Here's how the part is built. I have some questions about the finished solid (model axes, mm). Give positions to 0.01 mm unless a question says otherwise; leave off trailing zeros. Order: outer loops, then holes, each group sorted by start corner. A loop starts at its lowest first (then second) coordinate and runs counter-clockwise, first axis right, second up. Notation, with made-up numbers: M -36.5,44.25 L -17.5,44.25 A27 cw -17.5,77.25 Z; hole C 34,1 d1. An arc over 180 degrees is marked long. Use one line per item in the form item = value.
from build123d import *

# Parameters (mm, degrees)
SKETCH1_R           = 2
BOSS_EXTRUDE1_DEPTH = 50


with BuildPart() as part:
    # Sketch1 → Boss-Extrude1 (new body)
    with BuildSketch(Plane.XY):
        with BuildLine():
            Line((3.9, 2.839339828), (5.451585007, 4.390924835))
            ThreePointArc((5.451585007, 4.390924835), (4.949747468, 4.949747468), (4.390924835, 5.451585007))
            Line((4.390924835, 5.451585007), (2.839339828, 3.9))
            Line((2.839339828, 3.9), (0.519615242, 3.9))
            Line((0.519615242, 3.9), (0, 3.6))
            Line((0, 3.6), (-0.519615242, 3.9))
            Line((-0.519615242, 3.9), (-2.839339828, 3.9))
            Line((-2.839339828, 3.9), (-4.390924835, 5.451585007))
            ThreePointArc((-4.390924835, 5.451585007), (-4.949747468, 4.949747468), (-5.451585007, 4.390924835))
            Line((-5.451585007, 4.390924835), (-3.9, 2.839339828))
            Line((-3.9, 2.839339828), (-3.9, 0.519615242))
            Line((-3.9, 0.519615242), (-3.6, 0))
            Line((-3.6, 0), (-3.9, -0.519615242))
            Line((-3.9, -0.519615242), (-3.9, -2.839339828))
            Line((-3.9, -2.839339828), (-5.451585007, -4.390924835))
            ThreePointArc((-5.451585007, -4.390924835), (-4.949747468, -4.949747468), (-4.390924835, -5.451585007))
            Line((-4.390924835, -5.451585007), (-2.839339828, -3.9))
            Line((-2.839339828, -3.9), (-0.519615242, -3.9))
            Line((-0.519615242, -3.9), (0, -3.6))
            Line((0, -3.6), (0.519615242, -3.9))
            Line((0.519615242, -3.9), (2.839339828, -3.9))
            Line((2.839339828, -3.9), (4.390924835, -5.451585007))
            ThreePointArc((4.390924835, -5.451585007), (4.949747468, -4.949747468), (5.451585007, -4.390924835))
            Line((5.451585007, -4.390924835), (3.9, -2.839339828))
            Line((3.9, -2.839339828), (3.9, -0.519615242))
            Line((3.9, -0.519615242), (3.6, 0))
            Line((3.6, 0), (3.9, 0.519615242))
            Line((3.9, 0.519615242), (3.9, 2.839339828))
        make_face()
        Circle(SKETCH1_R, mode=Mode.SUBTRACT)
    extrude(amount=BOSS_EXTRUDE1_DEPTH)


solid = part.part
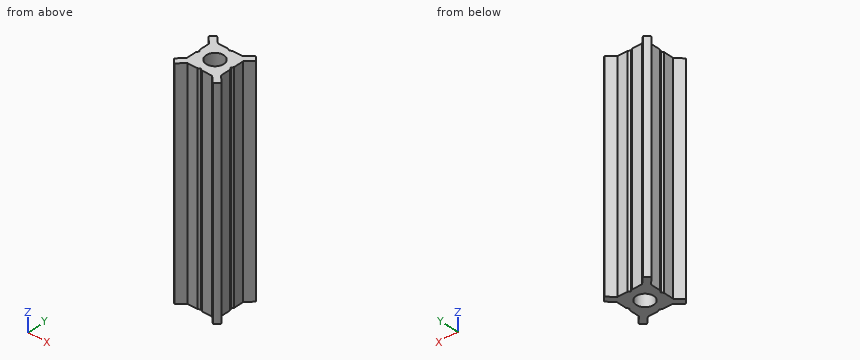
Q1. I'm going to push flat-ended pins straight in: pin 1 Ø1.2 at (x, z) = (-1.5, 16) entering from -Y; pin 2 Ø0.7 at (y, z) = (-1.5, 33.5) entering from -X; pin 3 Ø1.2 at (x, z) = (1.5, 14.5) entering from +Y; pin 4 Ø2.5 at (x, y) = (0, 0) entering from +Z. Where does each tip first touch, or does it pass through?
Found:
pin_1 = -3.9
pin_2 = -3.9
pin_3 = 3.9
pin_4 = through
Q2. I want a section at B-B on x = -1.25. Write out the boundary of the cut face in (y, z), then the cut area to 3 significant figures.
Found:
outline = M -3.9,0 L -1.56,0 L -1.56,50 L -3.9,50 Z; M 1.56,0 L 3.9,0 L 3.9,50 L 1.56,50 Z
area = 234 mm²
Q3. I need wall thicknesses on L1, parallel to Y at x = 0, z = 24.5; L2, parallel to Y at x = 2.5, z = 21; L3, parallel to X at y = -1.25, z = 22. Which ranges of each line are inside material? Lowest first, please.
Found:
L1 = -3.6 to -2, 2 to 3.6
L2 = -3.9 to 3.9
L3 = -3.9 to -1.56, 1.56 to 3.9
